Autodesk Inventor part; units mm, degrees
ref_plane "YZ Plane" through (0, 0, 0) normal (1, 0, 0) x (0, 1, 0)
ref_plane "XZ Plane" through (0, 0, 0) normal (0, 1, 0) x (-1, 0, 0)
ref_plane "XY Plane" through (0, 0, 0) normal (0, 0, 1) x (1, 0, 0)
sketch "Sketch1" plane through (0, 0, 0) normal (0, 0, 1) x (1, 0, 0)
  circle A0 centre (0, 0) radius 75
  line L0 (15, 73.4847) -> (15, -73.4847)
  line L1 (-15, -73.4847) -> (-15, 73.4847)
  dimension "d0" = 150
  dimension "d2" = 15
extrude "Extrusion1" add sketch "Sketch1" against normal blind 16 contours L0 A0 L1
sketch "Sketch2" plane through (0, 0, 0) normal (0, 0, 1) x (1, 0, 0)
  circle A0 centre (0, 0) radius 75
extrude "Extrusion2" add sketch "Sketch2" along normal blind 32
sketch "Sketch3" plane through (0, 0, 32) normal (0, 0, 1) x (1, 0, 0)
  line L0 (-75, 15) -> (75, 15)
  line L1 (75, 15) -> (75, -15)
  line L2 (75, -15) -> (-75, -15)
  line L3 (-75, -15) -> (-75, 15)
  point P0 (0, 0)
  dimension "d7" = 30
  dimension "d8" = 15
  dimension "d9" = 75
  dimension "d10" = 75
extrude "Extrusion3" cut sketch "Sketch3" along normal blind 32
sketch "Sketch4" plane through (0, 0, 32) normal (0, 0, 1) x (1, 0, 0)
  line L0 (-73.4847, 15) -> (73.4847, 15)
  line L1 (73.4847, -15) -> (-73.4847, -15)
  arc A0 (-73.4847, 15) -> (-73.4847, -15) centre (0, 0) ccw
  arc A1 (73.4847, -15) -> (73.4847, 15) centre (0, 0) ccw
extrude "Extrusion4" add sketch "Sketch4" along normal blind 16
CAD build for the part. Positions are in the model's coordinates, mm. A direction names the side the tool comes from. Round coordinates to 2 decimals unless told otherwise and drop trailing zeros. Loops run counter-clockwise (first coordinate to the right, second up) from the corner with the lowest first, then second, coordinate; pieces in that order, holes last. Notation, with made-up numbers: (59, 66.25) - (73, 66.25) arc R25 cw to (73, 85.25) - close; hole circle Ø2 at (49, 73.25). An arc over 180 degrees is marked (long way). Put each result on its own line as item: value.
1. Pin check, flat tips, straight feed: P1, Ø8, axis at x = 17.5, z = 37.5, coming from the +Y side; P2, Ø10, axis at x = -40, z = 5, coming from the -Y side; P3, Ø5, axis at y = -8, z = -10, coming from the -X side. Stop position of each tip, or through.
Geometry check:
P1: y = 15
P2: y = -66.33
P3: x = -15
2. Slice it at D-D on y = 19. List the corners of the cut face in (x, z), and give its area (3 significant figures).
Geometry check:
outline: (-72.55, 0) - (-15, 0) - (-15, -16) - (15, -16) - (15, 0) - (72.55, 0) - (72.55, 32) - (-72.55, 32) - close
area: 5,120 mm²
3. Wall check: line 1 (Z direction, x = -44, y = -31); line 2 (X direction, y = -26, z = -2); line 3 (Z direction, x = -1, y = -64). Give the ranges that are in metal, low to high.
Geometry check:
line 1: 0 to 32
line 2: -15 to 15
line 3: -16 to 32
4. Slice it at B-B on x = 0. List the corners of the cut face in (y, z), and give its area (3 significant figures).
Geometry check:
outline: (-75, -16) - (75, -16) - (75, 32) - (15, 32) - (15, 48) - (-15, 48) - (-15, 32) - (-75, 32) - close
area: 7,680 mm²
5. 3-axis set-ups, long thin cutter, end or side, ignore diameter. For faces 1 (the flat face through (-1, 39, 32)), 2 (the flat face through (-15, -1, -8)), 3 (the flat face through (38, 1, 0)), 4 (the flat face through (1, -15, 40)): which of +Z, -Z, +X, -X, +Y, -Y reach the whole face in a straight line?
Geometry check:
face 1: +Z, +X, -X, +Y
face 2: -Z, -X, +Y, -Y
face 3: -Z, +X, +Y, -Y
face 4: +Z, +X, -X, -Y
6. Slice it at C-C on z = -5. List the corners of the cut face in (x, y), and give its area (3 significant figures).
Geometry check:
outline: (-15, -73.48) arc R75 ccw to (15, -73.48) - (15, 73.48) arc R75 ccw to (-15, 73.48) - close
area: 4,470 mm²
7. Slice it at A-A on y = 0. List the corners of the cut face in (x, z).
Geometry check:
outline: (-75, 0) - (-15, 0) - (-15, -16) - (15, -16) - (15, 0) - (75, 0) - (75, 48) - (-75, 48) - close
